Design review of the part shown in the three views and the two pictorial views. Dimensions are in mm from the part's minimum x, y and z. A direction names the side the tool comes from. Round coordinates to 2 decimals unless told otherwise and drop trailing zeros. Write each loop counter-clockwise with the first axis right and the second up, starting at its lowest first coordinate (ties: lowest second). Pieces come first, ordered by that corner, then holes. Notation, with made-up numbers: (24, -7.5) - (35, -7.5) arc R23 ccw to (35, 11.5) - close; hole circle Ø4 at (25, -19.75). An arc over 180 degrees is marked (long way). Use one line per item in the form item = value.
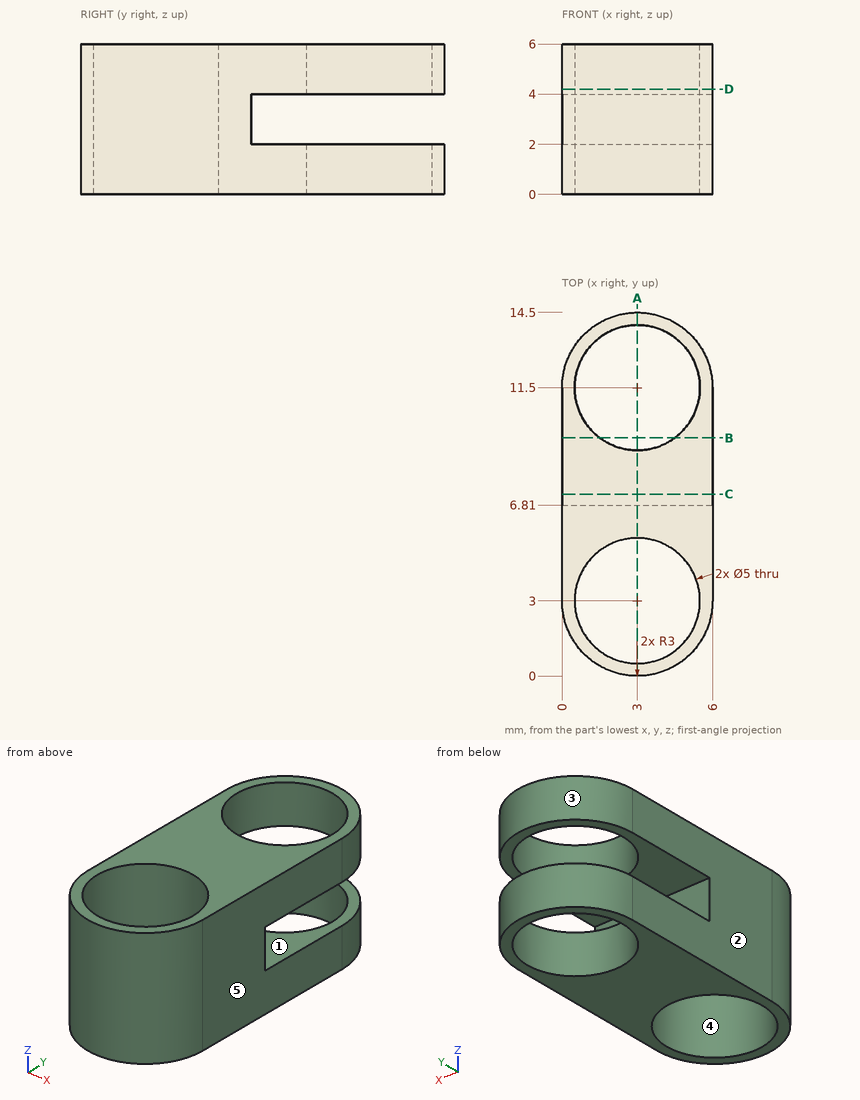
(1) The part is to be moulded in two halves that separate along Y. For the marked faces 3, 4 and 5, say which applies: +Y half, -Y half, draft (parallel to the pull), parting line (faces both ways), or undercut.
Geometry results:
face_3 = +Y half
face_4 = undercut
face_5 = draft
(2) Machinability: for the marked faces 1 and 2, which of the approach directions +Z, -Z, +X, -X, +Y, -Y give a long, thin tool a straight path to every point of the face, cutting with its end or side? Answer none if there is none.
Geometry results:
face_1 = +X, -X, +Y
face_2 = +Z, -Z, -X, +Y, -Y
(3) Add section A-A on x = 3. Write out the cut boundary in (y, z), then the cut area to 3 significant figures.
Geometry results:
outline = (0, 0) - (0.5, 0) - (0.5, 6) - (0, 6) - close; (5.5, 0) - (9, 0) - (9, 2) - (6.81, 2) - (6.81, 4) - (9, 4) - (9, 6) - (5.5, 6) - close; (14, 0) - (14.5, 0) - (14.5, 2) - (14, 2) - close; (14, 4) - (14.5, 4) - (14.5, 6) - (14, 6) - close
area = 21.6 mm2
(4) Add section B-B on y = 9.5. Write out the cut boundary in (x, z).
Geometry results:
outline = (0, 0) - (1.5, 0) - (1.5, 2) - (0, 2) - close; (0, 4) - (1.5, 4) - (1.5, 6) - (0, 6) - close; (4.5, 0) - (6, 0) - (6, 2) - (4.5, 2) - close; (4.5, 4) - (6, 4) - (6, 6) - (4.5, 6) - close
(5) Add section C-C on y = 7.25. Write out the cut boundary in (x, z).
Geometry results:
outline = (0, 0) - (6, 0) - (6, 2) - (0, 2) - close; (0, 4) - (6, 4) - (6, 6) - (0, 6) - close
(6) To check wall thickness, follow L1, parallel to Y at x = 3, z = 5.45; L2, parallel to Z at x = 0.4, y = 8.5; L3, parallel to Y at x = 4.9, z = 0.55 (1 decimal). State the ranges of each line that lie inside material, in increasing order.
Geometry results:
L1 = 0 to 0.5, 5.5 to 9, 14 to 14.5
L2 = 0 to 2, 4 to 6
L3 = 0.7 to 1.4, 4.6 to 9.9, 13.1 to 13.8
(7) Add section D-D on z = 4.2. Write out the cut boundary in (x, y).
Geometry results:
outline = (0, 3) arc R3 ccw to (6, 3) - (6, 11.5) arc R3 ccw to (0, 11.5) - close; hole circle Ø5 at (3, 3); hole circle Ø5 at (3, 11.5)
(8) Insertion check: P1, Ø1.5, axis at y = 8, z = 3.5, coming from the +X side; P2, Ø0.6, axis at x = 3, z = 2.5, coming from the +Y side; P3, Ø1, axis at x = 5, z = 4, coming from the +Y side. Each pin has a flat end and moves straight along its axis. Give the tip position at first contact, or say it passes through.
Geometry results:
P1 = 6
P2 = 6.81
P3 = 14.1
